```python
from build123d import *

# Parameters (mm, degrees)
BOSS_EXTRUDE2_DEPTH      = 38.1
BOSS_EXTRUDE2_DEPTH_BACK = 38.1
SKETCH3_R                = 3.175
CUT_EXTRUDE5_DEPTH       = 39.363670966
CUT_EXTRUDE5_DEPTH_BACK  = 39.363670966
SKETCH10_W               = 2.38125
SKETCH10_H               = 1.422321225
CHAMFER1_SIZE            = 0.3175


with BuildPart() as part:
    # Sketch3 → Boss-Extrude2 (new, two sides: drawn at the far end of the back side and taken through both)
    with BuildSketch(Plane.XY.offset(-BOSS_EXTRUDE2_DEPTH_BACK)):
        with Locations(Location((0, 0, 0), (0, 0, 180))):
            Circle(SKETCH3_R)
    extrude(amount=BOSS_EXTRUDE2_DEPTH + BOSS_EXTRUDE2_DEPTH_BACK)

    # Sketch10 → Cut-Extrude5 (cut, two sides: drawn at the far end of the back side and taken through both)
    with BuildSketch(Plane.XY.offset(-CUT_EXTRUDE5_DEPTH_BACK)):
        with Locations((0, 2.463839388)):
            Rectangle(SKETCH10_W, SKETCH10_H)
    extrude(amount=CUT_EXTRUDE5_DEPTH + CUT_EXTRUDE5_DEPTH_BACK, mode=Mode.SUBTRACT)

    # Chamfer1
    chamfer1_edges = [part.edges().sort_by_distance(p)[0] for p in [
        (0, -3.175, 38.1),
        (0, -3.175, -38.1),
    ]]
    chamfer(chamfer1_edges, length=CHAMFER1_SIZE)


solid = part.part
```
Input: part model. Units: mm. Frame: model coordinates. A direction names the side the tool comes from. Round coordinates to 2 decimals unless told otherwise and drop trailing zeros. Loops run counter-clockwise (first coordinate to the right, second up) from the corner with the lowest first, then second, coordinate; pieces in that order, holes last. Notation, with made-up numbers: (33.5, -1.75) - (70.5, -1.75) arc R16 cw to (70.5, 14.25) - close; hole circle Ø7 at (33, -21.5). An arc over 180 degrees is marked (long way). One line per item, written item: value. Start each with the question number.
(1) Section B-B, the plane z = 24.5. Return loops of the section in (x, y) (3 decimals), plus the area to 3 significant figures.
(2) Draft query along X for faces 3 (the conical face through (-0.115, -2.977, -37.979)), 4 (the flat face through (0, 1.753, -1)), 5 (the flat face through (0, 0, 38.1)). Return one class per face: +X half, -X half, draft (parallel to the pull), parting line (faces both ways), or undercut.
(3) Contact query for flat-ended pins moving along their axis: P1, Ø1, axis at x = 0, z = -6.5, coming from the +Y side; P2, Ø0.6, axis at y = 2.5, z = -6.5, coming from the +X side. Output: stop coordinate, or through.
(4) Ray query, line 1 (Y direction, x = 0, z = -27) (3 decimals); line 2 (X direction, y = 0.25, z = -3); line 3 (X direction, y = 2.5, z = -4). Return the intervals inside material, ascending. Write a range as [from, to].
(5) Access query for faces 1 (the flat face through (0, 0, -38.1)), 2 (the flat face through (1.191, 2, -1)). Directions: +Z, -Z, +X, -X, +Y, -Y. A direction counts if a zero-diameter tool reaches every point of the face in a straight line with its end or side. Return the directions, or none.
(6) Section A-A, the plane x = 0. Return loops of the section in (y, z) (1 decimal), plus the area to 3 significant figures.
Results below:
1. outline: (-1.191, 1.753) - (-1.191, 2.943) arc R3.175 ccw (long way) to (1.191, 2.943) - (1.191, 1.753) - close
1. area: 28.5 mm^2
2. face 3: parting line
2. face 4: undercut
2. face 5: draft
3. P1: y = 1.75
3. P2: x = 2.29
4. line 1: [-3.175, 1.753]
4. line 2: [-3.17, 3.17]
4. line 3: [-1.96, -1.19], [1.19, 1.96]
5. face 1: -Z, +X, -X, +Y, -Y
5. face 2: +Z, -Z, +Y
6. outline: (-3.2, -37.8) - (-2.9, -38.1) - (1.8, -38.1) - (1.8, 38.1) - (-2.9, 38.1) - (-3.2, 37.8) - close
6. area: 375 mm^2
